Verification items for the finished model (mm, model axes). Face numbers are marked on the shaded views. A direction names the side the tool comes from. Give positions to 0.01 mm unless a question says otherwise; leave off trailing zeros. Loops run counter-clockwise (first coordinate to the right, second up) from the corner with the lowest first, then second, coordinate; pieces in that order, holes last. Notation, with made-up numbers: (-27, -38.75) -> (-19, -38.75) arc R33 ccw to (-19, -0.75) -> close; hole circle Ø4 at (-31.5, 16.25). An arc over 180 degrees is marked (long way). Answer in a Markdown table with one row per item. Add a question column.
Q1. Set-up check for the marked faces 1, 2 and 3: record each of +Z, -Z, +X, -X, +Y, -Y from which the full face is reachable in a straight line by a thin tool's end or side.
Q2. Material ranges on probe 1 along Y at (x, z) = (-10, -11); probe 2 along Y at (x, z) = (-2, -2), recorded low to high.
Q3. Gauge pin test, flat ends, axial feed: P1, Ø2, axis at y = 2.5, z = 1, coming from the +X side; P2, Ø1.5, axis at y = -11, z = -7, coming from the -X side. Record the tip position at first contact, or that the pin passes through.
Q4. Section check D-D on z = 4.5. Enter the section's corners in (x, y), and give its area (3 significant figures).
Q5. Release check for a two-part mould opening along Y. For the marked faces 4, 5 and 6 record: pulls with the +Y half, pulls with the -Y half, needs draft (parallel to the pull), parting line crosses it, or undercut.
Q6. Section check A-A on y = -11. Enter the section's corners in (x, z), and give its area (3 significant figures).
Q7. Section check B-B on z = -4.5. Enter the section's corners in (x, y).
Q8. Section check C-C on x = 15. Enter the section's corners in (y, z).
```python
from build123d import *

# Parameters (mm, degrees)
SKETCH10_W          = 2.54
SKETCH10_H          = 5.08
SKETCH10_W_2        = 5.08
SKETCH10_H_2        = 2.54
BOSS_EXTRUDE3_DEPTH = 25.4
SKETCH11_W          = 31.4
SKETCH11_H          = 31.4
SKETCH11_W_2        = 25.4
SKETCH11_H_2        = 25.4
BOSS_EXTRUDE5_DEPTH = 25.4
BOSS_EXTRUDE6_DEPTH = 31.4


with BuildPart() as part:
    # Sketch10 → Boss-Extrude3 (new body)
    with BuildSketch(Plane(origin=(0, 0, 0), x_dir=(0, 0, -1), z_dir=(1, 0, 0))):
        with Locations((-11.43, 0)):
            Rectangle(SKETCH10_W, SKETCH10_H)
        with BuildLine():
            Line((-5.08, 2.54), (-9.740509205, 6.542688341))
            ThreePointArc((-9.740509205, 6.542688341), (-10.012022021, 6.580814495), (-10.16, 6.35))
            Line((-10.16, 6.35), (-10.16, -6.35))
            ThreePointArc((-10.16, -6.35), (-10.012022021, -6.580814495), (-9.740509205, -6.542688341))
            Line((-9.740509205, -6.542688341), (-5.08, -2.54))
            Line((-5.08, -2.54), (-5.08, 2.54))
        make_face()
        with BuildLine():
            Line((6.35, 10.16), (-6.35, 10.16))
            ThreePointArc((-6.35, 10.16), (-6.580814495, 10.012022021), (-6.542688341, 9.740509205))
            Line((-6.542688341, 9.740509205), (-2.54, 5.08))
            Line((-2.54, 5.08), (2.54, 5.08))
            Line((2.54, 5.08), (6.542688341, 9.740509205))
            ThreePointArc((6.542688341, 9.740509205), (6.580814495, 10.012022021), (6.35, 10.16))
        make_face()
        with Locations((0, 11.43)):
            Rectangle(SKETCH10_W_2, SKETCH10_H_2)
        with BuildLine():
            ThreePointArc((6.542688341, -9.740509205), (6.580814495, -10.012022021), (6.35, -10.16))
            Line((6.35, -10.16), (-6.35, -10.16))
            ThreePointArc((-6.35, -10.16), (-6.580814495, -10.012022021), (-6.542688341, -9.740509205))
            Line((-6.542688341, -9.740509205), (-2.54, -5.08))
            Line((-2.54, -5.08), (2.54, -5.08))
            Line((2.54, -5.08), (6.542688341, -9.740509205))
        make_face()
        with Locations((0, -11.43)):
            Rectangle(SKETCH10_W_2, SKETCH10_H_2)
        with BuildLine():
            Line((5.08, 2.54), (5.08, -2.54))
            Line((5.08, -2.54), (9.740509205, -6.542688341))
            ThreePointArc((9.740509205, -6.542688341), (10.012022021, -6.580814495), (10.16, -6.35))
            Line((10.16, -6.35), (10.16, -2.54))
            Line((10.16, -2.54), (10.16, 2.54))
            Line((10.16, 2.54), (10.16, 6.35))
            ThreePointArc((10.16, 6.35), (10.012022021, 6.580814495), (9.740509205, 6.542688341))
            Line((9.740509205, 6.542688341), (5.08, 2.54))
        make_face()
        with Locations((11.43, 0)):
            Rectangle(SKETCH10_W, SKETCH10_H)
    extrude(amount=-BOSS_EXTRUDE3_DEPTH)

    # Sketch11 → Boss-Extrude5 (add, through all)
    with BuildSketch(Plane(origin=(0, 0, 0), x_dir=(0, 0, -1), z_dir=(1, 0, 0))):
        Rectangle(SKETCH11_W, SKETCH11_H)
        Rectangle(SKETCH11_W_2, SKETCH11_H_2, mode=Mode.SUBTRACT)
    extrude(amount=-BOSS_EXTRUDE5_DEPTH)

    # Sketch13 → Boss-Extrude6 (add, through all)
    with BuildSketch(Plane.XZ.offset(15.7)):
        Polygon((0, 15.7), (12.7, 15.7), (12.7, -3.35), (19.05, -15.7), (0, -15.7), align=None)
    extrude(amount=-BOSS_EXTRUDE6_DEPTH)


solid = part.part
```
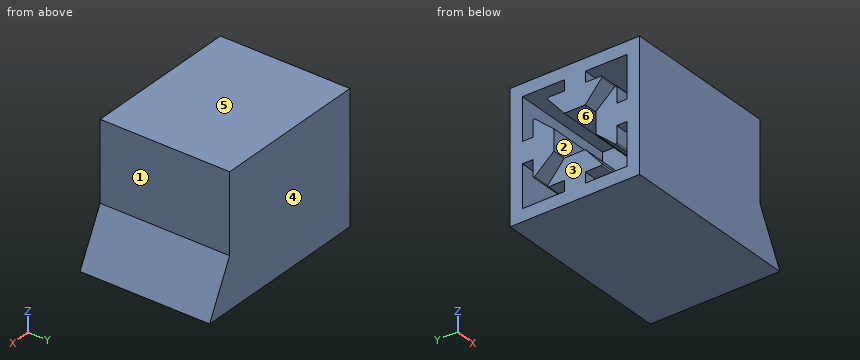
Taken from the geometry:
| question | item | result |
|---|---|---|
| 1 | face 1 | +Z, +X, +Y, -Y |
| 1 | face 2 | -X |
| 1 | face 3 | +Z, -Z, -X, +Y, -Y |
| 2 | probe 1 | y = -15.7 to -12.7, -2.54 to 2.54, 12.7 to 15.7 |
| 2 | probe 2 | y = -15.7 to -5.08, 5.08 to 15.7 |
| 3 | P1 | stops at x = 12.7 |
| 3 | P2 | stops at x = 0 |
| 4 | outline | (-25.4, -15.7) -> (12.7, -15.7) -> (12.7, 15.7) -> (-25.4, 15.7) -> (-25.4, 12.7) -> (0, 12.7) -> (0, 10.16) -> (-25.4, 10.16) -> (-25.4, 7.36) -> (0, 7.36) -> (0, -7.36) -> (-25.4, -7.36) -> (-25.4, -10.16) -> (0, -10.16) -> (0, -12.7) -> (-25.4, -12.7) -> close |
| 4 | area | 693 mm² |
| 5 | face 4 | pulls with the +Y half |
| 5 | face 5 | needs draft |
| 5 | face 6 | undercut |
| 6 | outline | (-25.4, -15.7) -> (19.05, -15.7) -> (12.7, -3.35) -> (12.7, 15.7) -> (-25.4, 15.7) -> (-25.4, 12.7) -> (0, 12.7) -> (0, 2.54) -> (-25.4, 2.54) -> (-25.4, -2.54) -> (0, -2.54) -> (0, -12.7) -> (-25.4, -12.7) -> close |
| 6 | area | 719 mm² |
| 7 | outline | (-25.4, -15.7) -> (13.29, -15.7) -> (13.29, 15.7) -> (-25.4, 15.7) -> (-25.4, 12.7) -> (0, 12.7) -> (0, 10.16) -> (-25.4, 10.16) -> (-25.4, 7.36) -> (0, 7.36) -> (0, -7.36) -> (-25.4, -7.36) -> (-25.4, -10.16) -> (0, -10.16) -> (0, -12.7) -> (-25.4, -12.7) -> close |
| 8 | outline | (-15.7, -15.7) -> (15.7, -15.7) -> (15.7, -7.82) -> (-15.7, -7.82) -> close |
